Work out the finished part from the listing and answer in its coordinate system (mm). Coordinates: 2 decimals unless noted, no trailing zeros. Order: outer loops, then holes, each group sorted by start corner. A loop starts at its lowest first (then second) coordinate and runs counter-clockwise, first axis right, second up. Notation, with made-up numbers: M 50.25,-11 L 58.25,-11 A25 cw 58.25,11 Z; hole C 13,26 d2. An arc over 180 degrees is marked long. Answer in a Markdown table with one row per item. Add a question column.
Item 1: Consider line 1 (X direction, y = 14, z = 6.4); line 2 (Y direction, x = 71.5, z = 5.6). Determine where each line is inside the solid, lowest interval first. Write a range as from..to.
Item 2: Flat-ended cylindrical pins translate along their axes: pin 1 Ø0.9 at (y, z) = (14.5, 7) entering from +X; pin 2 Ø1.5 at (x, z) = (25, 6.5) entering from +Y; pin 3 Ø1.5 at (y, z) = (6.5, 7) entering from -X; pin 4 Ø8 at (x, y) = (140, 33.5) entering from -Z. Find the tip coordinate at first contact, or state that the pin passes through.
Item 3: The part is cut by section B-B (z = 5.95). Write down the section's boundary in (x, y), then the cut area to 3 significant figures.
Item 4: The part is cut by section C-C (x = 21.5). Write down the section's boundary in (y, z).
Item 5: The part is cut by section A-A (y = 43.5). Write down the section's boundary in (x, z).
Autodesk Inventor part; units mm, degrees
ref_plane "Work Plane4" through (0, 0, 5) normal (0, 0, 1) x (1, 0, 0)
ref_plane "Work Plane8" through (0, 0, 5) normal (0, 0, 1) x (1, 0, 0)
ref_plane "Work Plane9" through (0, 0, 5) normal (0, 0, 1) x (1, 0, 0)
ref_plane "Work Plane4" through (0, 0, 5) normal (0, 0, 1) x (1, 0, 0)
sketch "Sketch2" plane through (0, 0, 5) normal (0, 0, 1) x (1, 0, 0)
  line L0 (0, 0) -> (235, 0)
  line L1 (235, 0) -> (235, 51)
  line L2 (235, 51) -> (0, 51)
  line L3 (0, 51) -> (0, 0)
  line L4 (235, 0) -> (235, 51)
  line L5 (0, 22.5) -> (235, 22.5)
  line L6 (235, 22.5) -> (235, 28.5)
  line L7 (235, 28.5) -> (0, 28.5)
  line L8 (0, 28.5) -> (0, 22.5)
  line L9 (0, 22.5) -> (235, 28.5) construction
  line L10 (235, 22.5) -> (0, 28.5) construction
  point P0 (117.5, 25.5)
  dimension "d4" = 6
extrude "Extrusion2" add sketch "Sketch2" along normal blind 3 contours L3 L7 L1 L5
ref_plane "Work Plane8" through (0, 0, 5) normal (0, 0, 1) x (1, 0, 0)
sketch "Sketch3" plane through (0, 0, 5) normal (0, 0, 1) x (1, 0, 0)
  line L0 (0, 28.5) -> (235, 28.5)
  line L1 (235, 51) -> (0, 51)
  line L2 (34.5, 28.5) -> (39.5, 28.5)
  line L3 (39.5, 28.5) -> (39.5, 51)
  line L4 (39.5, 51) -> (34.5, 51)
  line L5 (34.5, 51) -> (34.5, 28.5)
  point P0 (0, 0)
  dimension "d7" = 5
ref_plane "Work Plane9" through (0, 0, 5) normal (0, 0, 1) x (1, 0, 0)
sketch "Sketch5" plane through (0, 0, 5) normal (0, 0, 1) x (1, 0, 0)
  line L0 (235, 51) -> (0, 51)
  line L1 (117.5, 51) -> (117.5, 0)
  line L2 (235, 28.5) -> (0, 28.5)
  line L3 (34.5, 51) -> (39.5, 51)
  line L4 (39.5, 51) -> (39.5, 28.5)
  line L5 (39.5, 28.5) -> (34.5, 28.5)
  line L6 (34.5, 28.5) -> (34.5, 51)
  line L7 (0, 22.5) -> (235, 22.5)
  line L8 (34.5, 22.5) -> (39.5, 22.5)
  line L9 (39.5, 22.5) -> (39.5, 0)
  line L10 (39.5, 0) -> (34.5, 0)
  line L11 (34.5, 0) -> (34.5, 22.5)
  line L12 (195.5, 51) -> (195.5, 28.5)
  line L13 (200.5, 28.5) -> (200.5, 51)
  line L14 (195.5, 22.5) -> (195.5, 0)
  line L15 (195.5, 0) -> (200.5, 0)
  line L16 (200.5, 0) -> (200.5, 22.5)
  line L17 (195.5, 28.5) -> (200.5, 28.5)
  line L18 (195.5, 22.5) -> (200.5, 22.5)
  line L19 (195.5, 51) -> (200.5, 51)
  point P0 (0, 0)
  dimension "d13" = 5
extrude "Extrusion5" add sketch "Sketch3" along normal blind 3
extrude "Extrusion6" add sketch "Sketch5" along normal blind 3 contours L9 L10 L11 L7
extrude "Extrusion7" add sketch "Sketch5" along normal blind 3 contours L13 L2 L12 L0 | L7 L16 L15 L14
sketch "Sketch7" plane through (0, 0, 8) normal (0, 0, 1) x (1, 0, 0)
  line L0 (0, 28.5) -> (34.5, 28.5)
  line L1 (34.5, 28.5) -> (34.5, 51)
  line L2 (34.5, 51) -> (39.5, 51)
  line L3 (39.5, 51) -> (39.5, 28.5)
  line L4 (39.5, 28.5) -> (39.5, 51)
  line L5 (39.5, 28.5) -> (195.5, 28.5)
  line L6 (195.5, 28.5) -> (195.5, 51)
  line L7 (195.5, 51) -> (195.5, 28.5)
  line L8 (195.5, 51) -> (185.7081, 51)
  line L9 (200.5, 51) -> (200.5, 28.5)
  line L10 (200.5, 28.5) -> (200.5, 51)
  line L11 (200.5, 28.5) -> (235, 28.5)
  line L12 (235, 28.5) -> (235, 22.5)
  line L13 (235, 22.5) -> (200.5, 22.5)
  line L14 (200.5, 22.5) -> (200.5, 0)
  line L15 (200.5, 0) -> (200.5, 22.5)
  line L16 (200.5, 0) -> (195.5, 0)
  line L17 (195.5, 0) -> (200.5, 0)
  line L18 (195.5, 0) -> (195.5, 22.5)
  line L19 (195.5, 22.5) -> (39.5, 22.5)
  line L20 (0, 22.5) -> (235, 22.5)
  line L21 (39.5, 22.5) -> (39.5, 0)
  line L22 (39.5, 0) -> (34.5, 0)
  line L23 (34.5, 0) -> (39.5, 0)
  line L24 (34.5, 0) -> (34.5, 22.5)
  line L25 (34.5, 22.5) -> (34.5, 0)
  line L26 (34.5, 22.5) -> (0, 22.5)
  line L27 (0, 22.5) -> (0, 28.5)
  line L28 (0, 28.5) -> (0, 22.5)
  point P0 (0, 0)
properties part number "Brace" material "ABS Plastic"
Reply:
| question | item | result |
|---|---|---|
| 1 | line 1 | x = 34.5..39.5, 195.5..200.5 |
| 1 | line 2 | y = 22.5..28.5 |
| 2 | pin 1 | stops at x = 200.5 |
| 2 | pin 2 | stops at y = 28.5 |
| 2 | pin 3 | stops at x = 34.5 |
| 2 | pin 4 | passes through |
| 3 | outline | M 0,22.5 L 34.5,22.5 L 34.5,0 L 39.5,0 L 39.5,22.5 L 195.5,22.5 L 195.5,0 L 200.5,0 L 200.5,22.5 L 235,22.5 L 235,28.5 L 200.5,28.5 L 200.5,51 L 195.5,51 L 195.5,28.5 L 39.5,28.5 L 39.5,51 L 34.5,51 L 34.5,28.5 L 0,28.5 Z |
| 3 | area | 1,860 mm2 |
| 4 | outline | M 22.5,5 L 28.5,5 L 28.5,8 L 22.5,8 Z |
| 5 | outline | M 34.5,5 L 39.5,5 L 39.5,8 L 34.5,8 Z; M 195.5,5 L 200.5,5 L 200.5,8 L 195.5,8 Z |
